```python
from build123d import *

# Parameters (mm, degrees)
F1_DEPTH = 3
F2_D     = 7.5
F3_D     = 7


with BuildPart() as f1:
    # F0 (on Front) → F1 (new body)
    with BuildSketch(Plane.XZ):
        with BuildLine():
            ThreePointArc((44.3705983732, -77.5), (45.7264137346, -77.3126671094), (46.9806335717, -76.7647058824))
            ThreePointArc((46.9806335717, -76.7647058824), (89.9981580742, 0.57579792), (45.9945642101, 77.3595505618))
            ThreePointArc((45.9945642101, 77.3595505618), (45.7485129667, 77.4642485576), (45.4835134967, 77.5))
            Line((45.4835134967, 77.5), (44.5262354224, 77.5))
            ThreePointArc((44.5262354224, 77.5), (43.9102444687, 77.2877532259), (43.5557377006, 76.74111029))
            ThreePointArc((43.5557377006, 76.74111029), (43.0257432914, 68.0363839372), (45.6411198435, 59.7169512378))
            ThreePointArc((45.6411198435, 59.7169512378), (45.7279786025, 59.4899612828), (45.7575130443, 59.2487215672))
            Line((45.7575130443, 59.2487215672), (45.7575130443, 48.3390996312))
            ThreePointArc((45.7575130443, 48.3390996312), (45.9914686012, 47.6963120215), (46.5838648666, 47.3542918782))
            Line((46.5838648666, 47.3542918782), (52.6511673154, 46.2844627563))
            ThreePointArc((52.6511673154, 46.2844627563), (53.3983919294, 46.4501184651), (53.8096232461, 47.0956223317))
            Line((53.8096232461, 47.0956223317), (53.8964473349, 47.5880262082))
            ThreePointArc((53.8964473349, 47.5880262082), (54.3076786516, 48.2335300748), (55.0549032656, 48.3991857835))
            ThreePointArc((55.0549032656, 48.3991857835), (56.9914148655, 47.1654918335), (57.4883819916, 44.9238179915))
            Line((57.4883819916, 44.9238179915), (57.1410856363, 42.9542024855))
            ThreePointArc((57.1410856363, 42.9542024855), (55.9073916863, 41.0176908856), (53.6657178442, 40.5207237594))
            Line((53.6657178442, 40.5207237594), (49.7264868322, 41.2153164701))
            Line((49.7264868322, 41.2153164701), (49.813310921, 41.7077203466))
            ThreePointArc((49.813310921, 41.7077203466), (49.4819995036, 43.2021695746), (48.1909917703, 44.024632208))
            Line((48.1909917703, 44.024632208), (46.654928091, 44.2954816787))
            ThreePointArc((46.654928091, 44.2954816787), (45.3770547888, 44.0961843774), (44.4883207532, 43.1565932934))
            ThreePointArc((44.4883207532, 43.1565932934), (43.4498768152, 39.2184028407), (43.7884788704, 35.1597012623))
            ThreePointArc((43.7884788704, 35.1597012623), (44.0953044742, 34.5016388527), (44.6168439919, 33.9964808404))
            ThreePointArc((44.6168439919, 33.9964808404), (60.0850196139, 16.3699097283), (64.5841686774, -6.6456963673))
            ThreePointArc((64.5841686774, -6.6456963673), (64.5645764936, -6.784174398), (64.5258561915, -6.9185647133))
            Line((64.5258561915, -6.9185647133), (59.2200951601, -21.4309391015))
            ThreePointArc((59.2200951601, -21.4309391015), (59.1869810524, -21.540630442), (59.1666321841, -21.6533897337))
            ThreePointArc((59.1666321841, -21.6533897337), (52.1569189093, -38.7718630086), (37.4004437105, -49.9264426586))
            ThreePointArc((37.4004437105, -49.9264426586), (35.6386283719, -51.1165251582), (34.530567944, -52.9310476109))
            ThreePointArc((34.530567944, -52.9310476109), (33.3782658922, -64.5025194612), (37.5854765853, -75.34346679))
            ThreePointArc((37.5854765853, -75.34346679), (39.3763002237, -76.9281674511), (41.6982246465, -77.5))
            Line((41.6982246465, -77.5), (44.3705983732, -77.5))
        make_face()
        with BuildLine():
            ThreePointArc((56.8104775969, 58.0058225518), (58.0058225518, 60.5692480801), (60.5692480801, 59.3739031251))
            Line((60.5692480801, 59.3739031251), (63.3054092267, 51.8563621588))
            ThreePointArc((63.3054092267, 51.8563621588), (62.1100642717, 49.2929366306), (59.5466387435, 50.4882815855))
            Line((59.5466387435, 50.4882815855), (56.8104775969, 58.0058225518))
        make_face(mode=Mode.SUBTRACT)
        with BuildLine():
            ThreePointArc((72.1561451286, 17.555574771), (72.0027969224, 22.1492099685), (76.5964321199, 22.3025581748))
            Line((76.5964321199, 22.3025581748), (82.0737206627, 17.1791501079))
            ThreePointArc((82.0737206627, 17.1791501079), (82.2270688689, 12.5855149104), (77.6334336714, 12.4321667042))
            Line((77.6334336714, 12.4321667042), (72.1561451286, 17.555574771))
        make_face(mode=Mode.SUBTRACT)
    extrude(amount=F1_DEPTH)

    # F2 (through all)
    with Locations(Plane(origin=(0, 0, 0), x_dir=(1, 0, 0), z_dir=(0, 1, 0))):
        with Locations((67.5499814952, -39)):
            Hole(F2_D / 2)

    # F3 (through all)
    with Locations(Plane(origin=(0, 0, 0), x_dir=(1, 0, 0), z_dir=(0, 1, 0))):
        with Locations((77.7031864512, 6.7981479343), (62.8156443358, 52.7085839943)):
            Hole(F3_D / 2)


solid = f1.part
```
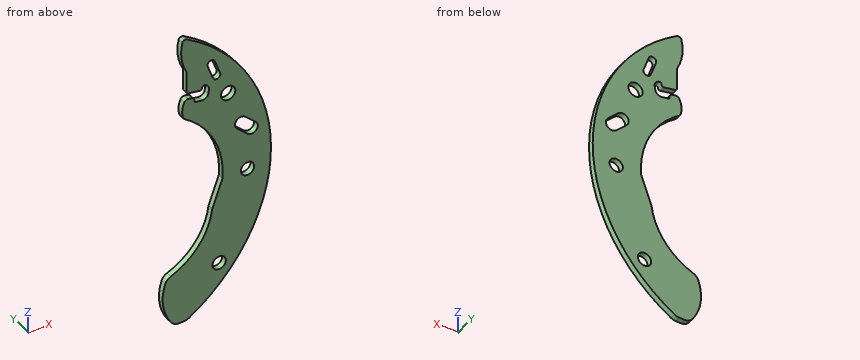
Source: CAD feature listing. Evaluate the final solid. Frame: model axes, mm. Round coordinates to 2 decimals unless told otherwise and drop trailing zeros. Loops run counter-clockwise (first coordinate to the right, second up) from the corner with the lowest first, then second, coordinate; pieces in that order, holes last.
1. Section query C-C on z = -37. Output: boundary loops of the cut face in (x, y).
2. Section query A-A on z = 39. Output: boundary loops of the cut face in (x, y), and give its area (3 significant figures).
3. Section query D-D on z = -19.5. Output: boundary loops of the cut face in (x, y).
4. Contact query for flat-ended pins moving along their axis: pin 1 (0.9 mm diameter, centred on y = -1.5, z = 53.5, fed in from -X); pin 2 (12 mm diameter, centred on x = 70.5, z = -56.5, fed in from +Y); pin 3 (4 mm diameter, centred on x = 62.82, z = -52.71, fed in from +Y). Output: stop coordinate, or through.
5. Section query B-B on y = -0.65. Give the number of separate pieces and of enclosed holes in the cut face, and give its area (3 significant figures).
6. Ray query, L1, parallel to Z at x = 46.5, y = -1.55; L2, parallel to Z at x = 79, y = -1.45; L3, parallel to X at y = -0.4, z = 38.5. Return the intervals inside material, ascending.
Answers below:
1. outline: (53.43, -3) - (82.04, -3) - (82.04, 0) - (53.43, 0) - close
2. outline: (43.43, -3) - (63.8, -3) - (63.8, 0) - (43.43, 0) - close; (71.3, -3) - (81.11, -3) - (81.11, 0) - (71.3, 0) - close
2. area: 90.5 mm2
3. outline: (59.93, -3) - (87.86, -3) - (87.86, 0) - (59.93, 0) - close
4. pin 1: stops at x = 45.76
4. pin 2: stops at y = 0
4. pin 3: passes through
5. separate pieces: 1
5. enclosed holes: 5
5. area: 3,930 mm2
6. L1: z = -77.02 to -44.58, 32.67 to 44.32, 47.37 to 77.06
6. L2: z = -43.12 to -10.05, -3.55 to 11.67, 20.05 to 43.12
6. L3: x = 43.41 to 63.83, 71.27 to 81.35
